from build123d import *

# Parameters (mm, degrees)
SKETCH1_W           = 15
SKETCH1_H           = 5
BOSS_EXTRUDE1_DEPTH = 5
CUT_EXTRUDE1_DEPTH  = 5
SKETCH3_R           = 2.1
CUT_EXTRUDE2_DEPTH  = 5
BOSS_EXTRUDE2_DEPTH = 5
SKETCH5_R           = 2.1
CUT_EXTRUDE3_DEPTH  = 5
SKETCH7_R           = 2.1
SKETCH7_R_2         = 1.973564221
BOSS_EXTRUDE3_DEPTH = 5
SKETCH8_R           = 2.1
CUT_EXTRUDE5_DEPTH  = 5
BOSS_EXTRUDE4_DEPTH = 5
SKETCH10_R          = 2
CUT_EXTRUDE6_DEPTH  = 10
SKETCH11_W          = 5
SKETCH11_H          = 5
BOSS_EXTRUDE5_DEPTH = 0.1
SKETCH12_W          = 5
SKETCH12_H          = 5
BOSS_EXTRUDE6_DEPTH = 0.1


with BuildPart() as part:
    # Sketch1 → Boss-Extrude1 (new body)
    with BuildSketch(Plane.XY):
        Polygon((-72.5, 0), (0, 0), (0, 140), (-35, 140), (-35, 145), (0, 145), (0, 155), (-35, 155), (-35, 160), (0, 160), (0, 170), (-35, 170), (-35, 175), (0, 175), (0, 185), (-35, 185), (-35, 190), (0, 190), (0, 245), (-30, 245), (-30, 250), (-55, 250), (-55, 245), (-115, 245), (-115, 250), (-140, 250), (-140, 245), (-170, 245), (-170, 190), (-135, 190), (-135, 185), (-170, 185), (-170, 175), (-135, 175), (-135, 170), (-170, 170), (-170, 160), (-135, 160), (-135, 155), (-170, 155), (-170, 145), (-135, 145), (-135, 140), (-170, 140), (-170, 0), (-97.5, 0), (-97.5, -5), (-72.5, -5), align=None)
        with Locations((-117.5, 202.5)):
            Rectangle(SKETCH1_W, SKETCH1_H, mode=Mode.SUBTRACT)
        with Locations((-52.5, 202.5)):
            Rectangle(SKETCH1_W, SKETCH1_H, mode=Mode.SUBTRACT)
    extrude(amount=BOSS_EXTRUDE1_DEPTH)

    # Sketch2 → Cut-Extrude1 (cut)
    with BuildSketch(Plane.XY.offset(5)):
        with BuildLine():
            Line((-123.169872981, 0), (-131.830127019, 0))
            ThreePointArc((-131.830127019, 0), (-127.5, 2.5), (-123.169872981, 0))
        make_face()
        with BuildLine():
            Line((-46.830127019, 0), (-38.169872981, 0))
            ThreePointArc((-38.169872981, 0), (-42.5, 2.5), (-46.830127019, 0))
        make_face()
    extrude(amount=-CUT_EXTRUDE1_DEPTH, mode=Mode.SUBTRACT)

    # Sketch3 → Cut-Extrude2 (cut)
    with BuildSketch(Plane.XY.offset(5)):
        with Locations((-85, -2.5)):
            Circle(SKETCH3_R)
    extrude(amount=-CUT_EXTRUDE2_DEPTH, mode=Mode.SUBTRACT)

    # Sketch4 → Boss-Extrude2 (add)
    with BuildSketch(Plane.XY.offset(5)):
        with BuildLine():
            Line((-89.330127019, -5), (-80.669872981, -5))
            ThreePointArc((-80.669872981, -5), (-85, -7.5), (-89.330127019, -5))
        make_face()
    extrude(amount=-BOSS_EXTRUDE2_DEPTH)

    # Sketch5 → Cut-Extrude3 (cut)
    with BuildSketch(Plane.XY.offset(5)):
        with Locations((-85, 202.5)):
            Circle(SKETCH5_R)
    extrude(amount=-CUT_EXTRUDE3_DEPTH, mode=Mode.SUBTRACT)

    # Sketch7 → Boss-Extrude3 (add)
    with BuildSketch(Plane.XY.offset(5)):
        with BuildLine():
            Line((-55, 0), (-55, -5))
            Line((-55, -5), (-80.669872981, -5))
            ThreePointArc((-80.669872981, -5), (-85, -7.5), (-89.330127019, -5))
            Line((-89.330127019, -5), (-115, -5))
            Line((-115, -5), (-115, 0))
            Line((-115, 0), (-123.169872981, 0))
            ThreePointArc((-123.169872981, 0), (-127.5, 2.5), (-131.830127019, 0))
            Line((-131.830127019, 0), (-170, 0))
            Line((-170, 0), (-170, -22.5))
            Line((-170, -22.5), (-155, -22.5))
            Line((-155, -22.5), (-155, -27.5))
            Line((-155, -27.5), (-143.770676698, -27.5))
            ThreePointArc((-143.770676698, -27.5), (-140, -29.21640483), (-136.229323302, -27.5))
            Line((-136.229323302, -27.5), (-125, -27.5))
            Line((-125, -27.5), (-125, -22.5))
            Line((-125, -22.5), (-89.330127019, -22.5))
            ThreePointArc((-89.330127019, -22.5), (-85, -20), (-80.669872981, -22.5))
            Line((-80.669872981, -22.5), (-45, -22.5))
            Line((-45, -22.5), (-45, -27.5))
            Line((-45, -27.5), (-33.770676698, -27.5))
            ThreePointArc((-33.770676698, -27.5), (-30, -29.21640483), (-26.229323302, -27.5))
            Line((-26.229323302, -27.5), (-15, -27.5))
            Line((-15, -27.5), (-15, -22.5))
            Line((-15, -22.5), (0, -22.5))
            Line((0, -22.5), (0, 0))
            Line((0, 0), (-38.169872981, 0))
            ThreePointArc((-38.169872981, 0), (-42.5, 2.5), (-46.830127019, 0))
            Line((-46.830127019, 0), (-55, 0))
        make_face()
        with Locations((-42.5, -2.5)):
            Circle(SKETCH7_R, mode=Mode.SUBTRACT)
        with Locations((-30, -24.21640483)):
            Circle(SKETCH7_R_2, mode=Mode.SUBTRACT)
        with Locations((-140, -24.21640483)):
            Circle(SKETCH7_R_2, mode=Mode.SUBTRACT)
        with Locations((-127.5, -2.5)):
            Circle(SKETCH7_R, mode=Mode.SUBTRACT)
    extrude(amount=-BOSS_EXTRUDE3_DEPTH)

    # Sketch8 → Cut-Extrude5 (cut)
    with BuildSketch(Plane.XY.offset(5)):
        with Locations((-42.5, 247.5)):
            Circle(SKETCH8_R)
        with Locations((-127.5, 247.5)):
            Circle(SKETCH8_R)
    extrude(amount=-CUT_EXTRUDE5_DEPTH, mode=Mode.SUBTRACT)

    # Sketch9 → Boss-Extrude4 (add)
    with BuildSketch(Plane.XY.offset(5)):
        with BuildLine():
            Line((-46.830127019, 250), (-38.169872981, 250))
            ThreePointArc((-38.169872981, 250), (-42.5, 252.5), (-46.830127019, 250))
        make_face()
        with BuildLine():
            Line((-123.169872981, 250), (-131.830127019, 250))
            ThreePointArc((-131.830127019, 250), (-127.5, 252.5), (-123.169872981, 250))
        make_face()
    extrude(amount=-BOSS_EXTRUDE4_DEPTH)

    # Sketch10 → Cut-Extrude6 (cut)
    with BuildSketch(Plane.XY.offset(5)):
        with Locations((-80.5, 22.5)):
            Circle(SKETCH10_R)
        with Locations((-80.5, 62.5)):
            Circle(SKETCH10_R)
        with Locations((-80.5, 102.5)):
            Circle(SKETCH10_R)
        with Locations((-80.5, 142.5)):
            Circle(SKETCH10_R)
        with Locations((-80.5, 182.5)):
            Circle(SKETCH10_R)
        with Locations((-80.5, 222.5)):
            Circle(SKETCH10_R)
        with Locations((-89.5, 222.5)):
            Circle(SKETCH10_R)
        with Locations((-89.5, 182.5)):
            Circle(SKETCH10_R)
        with Locations((-89.5, 142.5)):
            Circle(SKETCH10_R)
        with Locations((-89.5, 102.5)):
            Circle(SKETCH10_R)
        with Locations((-89.5, 62.5)):
            Circle(SKETCH10_R)
        with Locations((-89.5, 22.5)):
            Circle(SKETCH10_R)
    extrude(amount=-CUT_EXTRUDE6_DEPTH, mode=Mode.SUBTRACT)

    # Sketch11 → Boss-Extrude5 (add)
    with BuildSketch(Plane.ZY.offset(45)):
        with Locations((2.5, -25)):
            Rectangle(SKETCH11_W, SKETCH11_H)
    extrude(amount=BOSS_EXTRUDE5_DEPTH)

    # Sketch12 → Boss-Extrude6 (add)
    with BuildSketch(Plane(origin=(-125, 0, 0), x_dir=(0, 0, -1), z_dir=(1, 0, 0))):
        with Locations((-2.5, -25)):
            Rectangle(SKETCH12_W, SKETCH12_H)
    extrude(amount=BOSS_EXTRUDE6_DEPTH)


solid = part.part
For this review, take the finished solid that the model builds, in its own axes (mm). A direction names the side the tool comes from. Round coordinates to 2 decimals unless told otherwise and drop trailing zeros. Write item = value, one per line. Start each with the question number.
1. For pin 1 Ø1.5 at (x, z) = (-136.5, 2.5) entering from +Y; pin 2 Ø1.5 at (x, z) = (-139, 1) entering from -Y; pin 3 Ø3 at (x, y) = (-80.5, 182.5) entering from -Z; pin 4 Ø1.5 at (x, z) = (-77, 2.5) entering from -Y, all flat-tipped, find the tip position at first contact; note any pin that passes through.
2. Wall thickness on L1, parallel to X at y = 202.5, z = 1.1; L2, parallel to Y at x = -42.5, z = 3.15; L3, parallel to Y at x = -114, z = 1.5: over which ranges is each line inside the solid? List them lowest first.
3. Consider section A-A on z = 3.8. Give the number of separate pieces and of enclosed holes in the cut face, plus the area to 3 significant figures.
4. Draft analysis for pull direction Y (two halves, no side actions). For faces 5 (the face through (0, 180, 2)), 6 (the face through (-15, 245, 2)), 7 (the face through (-35, 172, 2)), state which applies: released by +Y, released by -Y, zero draft, split by the parting line, or undercut.
5. For faces 1 (the face through (-97.5, -2, 2)), 2 (the face through (-136, 250, 2)), 3 (the face through (-15, -25, 3)), 4 (the face through (-152, 185, 2)), list the 3-axis set-ups (+Z, -Z, +X, -X, +Y, -Y) from which the entire face can be reached by the end or side of a thin tool; tool diameter is ignored.
Evaluation:
q1.pin_1 = 250
q1.pin_2 = -29.21
q1.pin_3 = through
q1.pin_4 = -22.5
q2.L1 = -170 to -125, -110 to -87.1, -82.9 to -60, -45 to 0
q2.L2 = -27.5 to -4.6, -0.4 to 245.4, 249.6 to 252.5
q2.L3 = -22.5 to -5, 0 to 200, 205 to 245
q3.separate_pieces = 1
q3.enclosed_holes = 24
q3.area = 44,100 mm2
q4.face_5 = zero draft
q4.face_6 = released by +Y
q4.face_7 = undercut
q5.face_1 = +Z, -Z
q5.face_2 = +Z, -Z, -X, +Y
q5.face_3 = +Z, -Z, +X, -Y
q5.face_4 = +Z, -Z, -X
